```python
from build123d import *

# Parameters (mm, degrees)
F0_R     = 7
F0_R_2   = 1.5
F1_DEPTH = 1.5
F2_DEPTH = 1


# Not quite as in the source:
# - a feature names something its author has since deleted; it is built from what else it names


with BuildPart() as f1:
    # F0 (on Front) → F1 (new body, symmetric)
    with BuildSketch(Plane.XZ):
        with Locations((-19.8327995853, -33.1064267996)):
            Circle(F0_R)
        with Locations((-19.8327995853, -33.1064267996)):
            Circle(F0_R_2, mode=Mode.SUBTRACT)
    extrude(amount=F1_DEPTH, both=True)

    # F0 (on Front) → F2 (join, symmetric)
    with BuildSketch(Plane.XZ):
        with BuildLine():
            ThreePointArc((-22.8327995853, -25.6902283125), (-19.8327995853, -41.1064267996), (-16.8327995853, -25.6902283125))
            Line((-16.8327995853, -25.6902283125), (-16.8327995853, 9.3097716875))
            Line((-16.8327995853, 9.3097716875), (-19.8327995853, 51.3097716875))
            Line((-19.8327995853, 51.3097716875), (-22.8327995853, 9.3097716875))
            Line((-22.8327995853, 9.3097716875), (-22.8327995853, -25.6902283125))
        make_face()
        with Locations((-19.8327995853, -33.1064267996)):
            Circle(F0_R, mode=Mode.SUBTRACT)
        with BuildLine():
            ThreePointArc((-21.8327995853, 3.9472361095), (-19.8327995853, 5.9472361095), (-17.8327995853, 3.9472361095))
            Line((-17.8327995853, 3.9472361095), (-17.8327995853, -20.1542899013))
            ThreePointArc((-17.8327995853, -20.1542899013), (-19.8327995853, -22.1542899013), (-21.8327995853, -20.1542899013))
            Line((-21.8327995853, -20.1542899013), (-21.8327995853, 3.9472361095))
        make_face(mode=Mode.SUBTRACT)
    extrude(amount=F2_DEPTH, both=True)


solid = f1.part
```
Design review of the part built by this model. Coordinates are the model's own, in mm. A direction names the side the tool comes from. Coordinates: 2 decimals unless noted, no trailing zeros. Order: outer loops, then holes, each group sorted by start corner. A loop starts at its lowest first (then second) coordinate and runs counter-clockwise, first axis right, second up. Notation, with made-up numbers: (55.5, 45.25) -> (82.5, 45.25) arc R18 ccw to (82.5, 51.25) -> close; hole circle Ø5 at (27, 54). An arc over 180 degrees is marked (long way). One line per item, written item: value. Start each with the question number.
Q1. Tool access review of faces 5 (the cylindrical face through (-19.877, 0.014, 5.947)), 6 (the flat face through (-20, 1.5, -31)), 7 (the cylindrical face through (-26.826, -1.254, -32.799)), 8 (the flat face through (-16.833, 0, -8)): name each direction out of +Z, -Z, +X, -X, +Y, -Y from which nothing blocks a thin tool from reaching the whole face with its end or side.
Q2. Insertion check: pin 1 Ø0.6 at (y, z) = (0.5, 0.5) entering from +X; pin 2 Ø4 at (x, z) = (-14, -5) entering from +Y; pin 3 Ø1.5 at (x, z) = (-26, -29.5) entering from -Y; pin 4 Ø5 at (x, z) = (-20.5, 23) entering from -Y. Each pin has a flat end and moves straight along its axis. Give the tip position at first contact, or say it passes through.
Q3. Take a section at D-D, the plane z = 15. State the section outline as (x, y) points, then the cut area to 3 significant figures.
Q4. Take a section at C-C, the plane x = -16. State the section outline as (y, z) points, then the cut area to 3 significant figures.
Q5. For probe 1 along X at (y, z) = (0.1, -1); probe 2 along Y at (x, z) = (-20.25, 21); probe 3 along Z at (x, y) = (-19.5, -1.35), list the stretches that pass through material, from the lowest coordinate up.
Q6. Take a section at A-A, the plane y = -0.3. State the section outline as (x, z) points.
Q7. Take a section at B-B, the plane z = -28. State the section outline as (x, y) points.
Q8. Mouldability with a two-part tool opening along X and no side actions: class faces 1 (the flat face through (-22.833, 0, -8)), 2 (the flat face through (-17.833, 0, -8)), 3 (the flat face through (-20, -1.5, -31)), 4 (the cylindrical face through (-26.826, 1.246, -32.799)) as pulls with the +X half, pulls with the -X half, needs draft (parallel to the pull), parting line crosses it, or undercut.
Values follow:
1. face 5: +Y, -Y
1. face 6: +Z, -Z, +X, -X, +Y
1. face 7: -Y
1. face 8: +Z, +X, +Y, -Y
2. pin 1: stops at x = -16.83
2. pin 2: passes through
2. pin 3: stops at y = -1.5
2. pin 4: stops at y = -1
3. outline: (-22.43, -1) -> (-17.24, -1) -> (-17.24, 1) -> (-22.43, 1) -> close
3. area: 10.4 mm2
4. outline: (-1.5, -38.96) -> (-1, -38.96) -> (-1, -40.13) -> (1, -40.13) -> (1, -38.96) -> (1.5, -38.96) -> (1.5, -27.25) -> (1, -27.25) -> (1, -26.08) -> (-1, -26.08) -> (-1, -27.25) -> (-1.5, -27.25) -> close
4. area: 39.8 mm2
5. probe 1: x = -22.83 to -21.83, -17.83 to -16.83
5. probe 2: y = -1 to 1
5. probe 3: z = -40.1 to -34.57, -31.64 to -26.11
6. outline: (-22.83, -25.69) arc R8 ccw (long way) to (-16.83, -25.69) -> (-16.83, 9.31) -> (-19.83, 51.31) -> (-22.83, 9.31) -> close; hole (-21.83, -20.15) arc R2 ccw to (-17.83, -20.15) -> (-17.83, 3.95) arc R2 ccw to (-21.83, 3.95) -> close; hole circle Ø3 at (-19.83, -33.11)
7. outline: (-25.99, -1) -> (-24.62, -1) -> (-24.62, -1.5) -> (-15.04, -1.5) -> (-15.04, -1) -> (-13.67, -1) -> (-13.67, 1) -> (-15.04, 1) -> (-15.04, 1.5) -> (-24.62, 1.5) -> (-24.62, 1) -> (-25.99, 1) -> close
8. face 1: pulls with the -X half
8. face 2: undercut
8. face 3: needs draft
8. face 4: parting line crosses it
